Read the model definition and answer for the solid it produces. Units are mm, in the model's axes. Give positions to 0.01 mm unless a question says otherwise; leave off trailing zeros. Order: outer loops, then holes, each group sorted by start corner. A loop starts at its lowest first (then second) coordinate and runs counter-clockwise, first axis right, second up. Notation, with made-up numbers: (-11.5, -30) - (26.5, -30) arc R25 cw to (26.5, -8) - close; hole circle Ø9 at (23, -21). An arc over 180 degrees is marked (long way). Use a Markdown table: item, result. Add a question column.
1. A flat-ended cylindrical pin translates along its axis: P1, Ø11.5, axis at x = 75, z = 0, coming from the -Y side. Find the tip coordinate at first contact, or state that the pin passes through.
2. Consider L1, parallel to Z at x = 75, y = -3.5; L2, parallel to Z at x = 64.5, y = -3.5; L3, parallel to Z at x = 40, y = -10.5. Determine where each line is inside the solid, lowest interval first.
3. A cutting plane is placed at A-A on y = -7.25. Determine the outline of the cut face in (x, z).
```python
from build123d import *

# Parameters (mm, degrees)
F1_DEPTH = 12


with BuildPart() as f1:
    # F0 (on Front) → F1 (new body)
    with BuildSketch(Plane.XZ):
        with BuildLine():
            ThreePointArc((83.920553, -83.901291), (84.716768, -82.869093), (85, -81.596627))
            Line((85, -81.596627), (85, -63.001752))
            Line((85, -63.001752), (85, -43.001752))
            Line((85, -43.001752), (85, -23.001752))
            Line((85, -23.001752), (85, 1.998248))
            Line((85, 1.998248), (85, 4.821038))
            ThreePointArc((85, 4.821038), (84.427981, 6.583113), (82.930062, 7.673228))
            Line((82.930062, 7.673228), (71.507298, 11.398042))
            Line((71.507298, 11.398042), (62, 14.498248))
            Line((62, 14.498248), (52.492702, 17.598454))
            Line((52.492702, 17.598454), (40.510952, 21.505546))
            ThreePointArc((40.510952, 21.505546), (38.980302, 21.874305), (37.410746, 21.998248))
            Line((37.410746, 21.998248), (-37.410746, 21.998248))
            ThreePointArc((-37.410746, 21.998248), (-38.980302, 21.874305), (-40.510952, 21.505546))
            Line((-40.510952, 21.505546), (-52.492702, 17.598454))
            Line((-52.492702, 17.598454), (-62, 14.498248))
            Line((-62, 14.498248), (-71.507298, 11.398042))
            Line((-71.507298, 11.398042), (-82.930062, 7.673228))
            ThreePointArc((-82.930062, 7.673228), (-84.427981, 6.583113), (-85, 4.821038))
            Line((-85, 4.821038), (-85, 1.998248))
            Line((-85, 1.998248), (-85, -23.001752))
            Line((-85, -23.001752), (-85, -43.001752))
            Line((-85, -43.001752), (-85, -63.001752))
            Line((-85, -63.001752), (-85, -81.596627))
            ThreePointArc((-85, -81.596627), (-84.716768, -82.869093), (-83.920553, -83.901291))
            Line((-83.920553, -83.901291), (-67.834403, -97.306416))
            ThreePointArc((-67.834403, -97.306416), (-66.935126, -97.822567), (-65.91385, -98.001752))
            Line((-65.91385, -98.001752), (65.91385, -98.001752))
            ThreePointArc((65.91385, -98.001752), (66.935126, -97.822567), (67.834403, -97.306416))
            Line((67.834403, -97.306416), (83.920553, -83.901291))
        make_face()
        with BuildLine():
            ThreePointArc((38.990151, 16.936276), (39.376448, 16.859172), (39.755476, 16.751897))
            Line((39.755476, 16.751897), (76.550103, 4.753649))
            ThreePointArc((76.550103, 4.753649), (77.942127, 4.042757), (79.046635, 2.936791))
            ThreePointArc((79.046635, 2.936791), (79.75569, 1.54383), (80, 0))
            Line((80, 0), (80, -56.821412))
            ThreePointArc((80, -56.821412), (79.809692, -58.187745), (79.253254, -59.450068))
            ThreePointArc((79.253254, -59.450068), (78.373045, -60.512289), (77.236068, -61.293548))
            Line((77.236068, -61.293548), (24.875388, -87.473888))
            ThreePointArc((24.875388, -87.473888), (24.34317, -87.702486), (23.788085, -87.867997))
            ThreePointArc((23.788085, -87.867997), (23.217583, -87.968201), (22.63932, -88.001752))
            Line((22.63932, -88.001752), (0, -88.001752))
            Line((0, -88.001752), (-22.63932, -88.001752))
            ThreePointArc((-22.63932, -88.001752), (-23.217583, -87.968201), (-23.788085, -87.867997))
            ThreePointArc((-23.788085, -87.867997), (-24.34317, -87.702486), (-24.875388, -87.473888))
            Line((-24.875388, -87.473888), (-77.236068, -61.293548))
            ThreePointArc((-77.236068, -61.293548), (-78.373045, -60.512289), (-79.253254, -59.450068))
            ThreePointArc((-79.253254, -59.450068), (-79.809692, -58.187745), (-80, -56.821412))
            Line((-80, -56.821412), (-80, 0))
            ThreePointArc((-80, 0), (-79.75569, 1.54383), (-79.046635, 2.936791))
            ThreePointArc((-79.046635, 2.936791), (-77.942127, 4.042757), (-76.550103, 4.753649))
            Line((-76.550103, 4.753649), (-39.755476, 16.751897))
            ThreePointArc((-39.755476, 16.751897), (-39.376448, 16.859172), (-38.990151, 16.936276))
            ThreePointArc((-38.990151, 16.936276), (-38.598983, 16.982731), (-38.205373, 16.998248))
            Line((-38.205373, 16.998248), (0, 16.998248))
            Line((0, 16.998248), (38.205373, 16.998248))
            ThreePointArc((38.205373, 16.998248), (38.598983, 16.982731), (38.990151, 16.936276))
        make_face(mode=Mode.SUBTRACT)
        with BuildLine():
            Line((76.550103, 4.753649), (39.755476, 16.751897))
            ThreePointArc((39.755476, 16.751897), (39.376448, 16.859172), (38.990151, 16.936276))
            ThreePointArc((38.990151, 16.936276), (38.598983, 16.982731), (38.205373, 16.998248))
            Line((38.205373, 16.998248), (0, 16.998248))
            Line((0, 16.998248), (-38.205373, 16.998248))
            ThreePointArc((-38.205373, 16.998248), (-38.598983, 16.982731), (-38.990151, 16.936276))
            ThreePointArc((-38.990151, 16.936276), (-39.376448, 16.859172), (-39.755476, 16.751897))
            Line((-39.755476, 16.751897), (-76.550103, 4.753649))
            ThreePointArc((-76.550103, 4.753649), (-72.063209, 4.046635), (-70, 0))
            ThreePointArc((-70, 0), (-75, -5), (-80, 0))
            Line((-80, 0), (-80, -56.821412))
            ThreePointArc((-80, -56.821412), (-75, -51.821412), (-70, -56.821412))
            ThreePointArc((-70, -56.821412), (-72.371344, -61.074666), (-77.236068, -61.293548))
            Line((-77.236068, -61.293548), (-24.875388, -87.473888))
            ThreePointArc((-24.875388, -87.473888), (-24.34317, -87.702486), (-23.788085, -87.867997))
            ThreePointArc((-23.788085, -87.867997), (-23.217583, -87.968201), (-22.63932, -88.001752))
            Line((-22.63932, -88.001752), (0, -88.001752))
            Line((0, -88.001752), (22.63932, -88.001752))
            ThreePointArc((22.63932, -88.001752), (23.217583, -87.968201), (23.788085, -87.867997))
            ThreePointArc((23.788085, -87.867997), (24.34317, -87.702486), (24.875388, -87.473888))
            Line((24.875388, -87.473888), (77.236068, -61.293548))
            ThreePointArc((77.236068, -61.293548), (70.746746, -54.192757), (80, -56.821412))
            Line((80, -56.821412), (80, 0))
            ThreePointArc((80, 0), (70.953365, -2.936791), (76.550103, 4.753649))
        make_face()
    extrude(amount=F1_DEPTH)


solid = f1.part
```
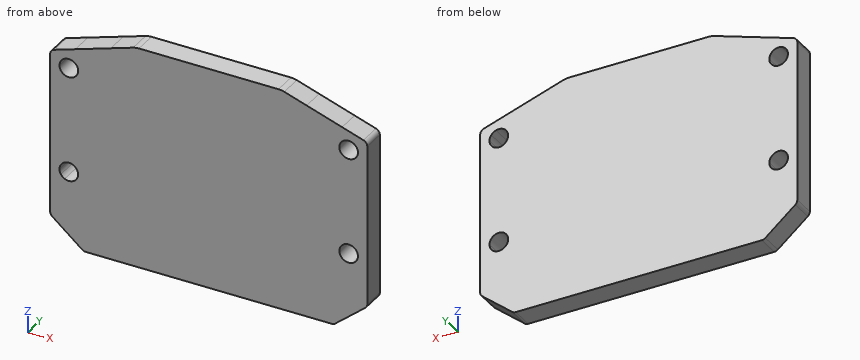
Output values:
| question | item | result |
|---|---|---|
| 1 | P1 | y = -12 |
| 2 | L1 | -91.34 to -61.82, -51.82 to -5, 5 to 10.26 |
| 2 | L2 | -98 to 13.68 |
| 2 | L3 | -98 to 21.66 |
| 3 | outline | (-85, -81.6) arc R3 ccw to (-83.92, -83.9) - (-67.83, -97.31) arc R3 ccw to (-65.91, -98) - (65.91, -98) arc R3 ccw to (67.83, -97.31) - (83.92, -83.9) arc R3 ccw to (85, -81.6) - (85, 4.82) arc R3 ccw to (82.93, 7.67) - (40.51, 21.51) arc R10 ccw to (37.41, 22) - (-37.41, 22) arc R10 ccw to (-40.51, 21.51) - (-82.93, 7.67) arc R3 ccw to (-85, 4.82) - close; hole (-80, -56.82) arc R5 ccw to (-79.25, -59.45) arc R5 ccw to (-77.24, -61.29) arc R5 ccw (long way) to start; hole (-79.05, 2.94) arc R5 ccw (long way) to (-70, 0) arc R5 ccw to (-76.55, 4.75) arc R5 ccw to start; hole (76.55, 4.75) arc R5 ccw (long way) to (79.05, 2.94) arc R5 ccw to start; hole (77.24, -61.29) arc R5 ccw to (79.25, -59.45) arc R5 ccw to (80, -56.82) arc R5 ccw (long way) to start |
